Verification items for the finished model (mm, model axes). A direction names the side the tool comes from. Round coordinates to 2 decimals unless told otherwise and drop trailing zeros. Write item = value, one per line. Start each with the question number.
from build123d import *

# Parameters (mm, degrees)
SKETCH1_R                        = 45.085
BOSS_EXTRUDE1_DEPTH              = 9.525
SKETCH2_R                        = 41.402
BOSS_EXTRUDE2_DEPTH              = 7.1374
SKETCH3_R                        = 45.085
BOSS_EXTRUDE3_DEPTH              = 3.175
SKETCH4_R                        = 41.529
BOSS_EXTRUDE4_DEPTH              = 7.1374
SKETCH5_R                        = 45.085
BOSS_EXTRUDE5_DEPTH              = 3.175
CIRPATTERN1_COUNT                = 8
M10X1_0_TAPPED_HOLE1_D           = 9
M10X1_0_TAPPED_HOLE1_DEPTH       = 25
M10X1_0_TAPPED_HOLE1_CBORE_D     = 10
M10X1_0_TAPPED_HOLE1_CBORE_DEPTH = 20
M10X1_0_TAPPED_HOLE1_TIP         = 2.703872786
SKETCH9_R                        = 32.259
CUT_EXTRUDE1_DEPTH               = 21.2598
SKETCH11_R                       = 50.546
BOSS_EXTRUDE6_DEPTH              = 9.525
SKETCH12_R                       = 28.575
CUT_EXTRUDE2_DEPTH               = 9.525
F_15_0_18_DIAMETER_HOLE1_D       = 4.572
F_15_0_18_DIAMETER_HOLE1_DEPTH   = 9.525
CIRPATTERN2_COUNT                = 8


with BuildPart() as part:
    # Sketch1 → Boss-Extrude1 (new body)
    with BuildSketch(Plane(origin=(0, 0, 0), x_dir=(1, 0, 0), z_dir=(0, 1, 0))):
        with Locations(Location((0, 0, 0), (0, 0, 90))):
            Circle(SKETCH1_R)
    extrude(amount=BOSS_EXTRUDE1_DEPTH)

    # Sketch2 → Boss-Extrude2 (add)
    with BuildSketch(Plane(origin=(0, 9.525, 0), x_dir=(1, 0, 0), z_dir=(0, 1, 0))):
        with Locations(Location((0, 0, 0), (0, 0, 270))):
            Circle(SKETCH2_R)
    extrude(amount=BOSS_EXTRUDE2_DEPTH)

    # Sketch3 → Boss-Extrude3 (add)
    with BuildSketch(Plane(origin=(0, 16.6624, 0), x_dir=(1, 0, 0), z_dir=(0, 1, 0))):
        with Locations(Location((0, 0, 0), (0, 0, 90))):
            Circle(SKETCH3_R)
    extrude(amount=BOSS_EXTRUDE3_DEPTH)

    # Sketch4 → Boss-Extrude4 (add)
    with BuildSketch(Plane(origin=(0, 19.8374, 0), x_dir=(1, 0, 0), z_dir=(0, 1, 0))):
        with Locations(Location((0, 0, 0), (0, 0, 270))):
            Circle(SKETCH4_R)
    extrude(amount=BOSS_EXTRUDE4_DEPTH)

    # Sketch5 → Boss-Extrude5 (add)
    with BuildSketch(Plane(origin=(0, 26.9748, 0), x_dir=(1, 0, 0), z_dir=(0, 1, 0))):
        with Locations(Location((0, 0, 0), (0, 0, 90))):
            Circle(SKETCH5_R)
    extrude(amount=BOSS_EXTRUDE5_DEPTH)

    # Sketch6 → #15 (0.18) Diameter Hole2 (revolve, cut)
    with BuildSketch(Plane(origin=(-45.085, 4.7625, 0), x_dir=(0, 0, 1), z_dir=(0, 1, 0))):
        Polygon((0, 0), (0, 6.373567375), (2.286, 5), (2.286, 0), align=None)
    f_15_0_18_diameter_hole2 = revolve(axis=Axis((-51.435, 4.7625, 0), (1, 0, 0)), mode=Mode.SUBTRACT)

    # CirPattern1: #15 (0.18) Diameter Hole2 ×8 about axis
    cirpattern1_axis = Axis((0, 9.525, 0), (0, -1, 0))
    for i in range(1, CIRPATTERN1_COUNT):
        add(f_15_0_18_diameter_hole2.rotate(cirpattern1_axis, i * 360 / CIRPATTERN1_COUNT), mode=Mode.SUBTRACT)

    # M10x1.0 Tapped Hole1
    with Locations(Plane(origin=(0, 0, 0), x_dir=(-1, 0, 0), z_dir=(0, -1, 0))):
        with Locations((0, 0)):
            CounterBoreHole(M10X1_0_TAPPED_HOLE1_D / 2, M10X1_0_TAPPED_HOLE1_CBORE_D / 2, M10X1_0_TAPPED_HOLE1_CBORE_DEPTH, depth=M10X1_0_TAPPED_HOLE1_DEPTH)
            with Locations((0, 0, -(M10X1_0_TAPPED_HOLE1_DEPTH + M10X1_0_TAPPED_HOLE1_TIP / 2))):  # 118° drill point
                Cone(0, M10X1_0_TAPPED_HOLE1_D / 2, M10X1_0_TAPPED_HOLE1_TIP, mode=Mode.SUBTRACT)

    # Sketch9 → Cut-Extrude1 (cut)
    with BuildSketch(Plane(origin=(0, 30.1498, 0), x_dir=(1, 0, 0), z_dir=(0, 1, 0))):
        with Locations(Location((0, 0, 0), (0, 0, 270))):
            Circle(SKETCH9_R)
    extrude(amount=-CUT_EXTRUDE1_DEPTH, mode=Mode.SUBTRACT)

    # Sketch11 → Boss-Extrude6 (add)
    with BuildSketch(Plane(origin=(0, 0, 0), x_dir=(-1, 0, 0), z_dir=(0, -1, 0))):
        with Locations(Location((0, 0, 0), (0, 0, 270))):
            Circle(SKETCH11_R)
    extrude(amount=BOSS_EXTRUDE6_DEPTH)

    # Sketch12 → Cut-Extrude2 (cut)
    with BuildSketch(Plane.XZ.offset(9.525)):
        with Locations(Location((0, 0, 0), (0, 0, 270))):
            Circle(SKETCH12_R)
    extrude(amount=-CUT_EXTRUDE2_DEPTH, mode=Mode.SUBTRACT)

    # #15 (0.18) Diameter Hole1
    with Locations(Plane(origin=(15.459601618, -9.525, -43.838083818), x_dir=(0, 0, -1), z_dir=(0, -1, 0))):
        with Locations((0, 0)):
            f_15_0_18_diameter_hole1 = Hole(F_15_0_18_DIAMETER_HOLE1_D / 2, depth=F_15_0_18_DIAMETER_HOLE1_DEPTH)

    # CirPattern2: #15 (0.18) Diameter Hole1 ×8 about axis
    cirpattern2_axis = Axis((0, 0, 0), (0, 1, 0))
    for i in range(1, CIRPATTERN2_COUNT):
        add(f_15_0_18_diameter_hole1.rotate(cirpattern2_axis, i * 360 / CIRPATTERN2_COUNT), mode=Mode.SUBTRACT)


solid = part.part
(1) Set-up check for faces 1 (the flat face through (45, 0, -8)), 2 (the cylindrical face through (19.36, -4.7, 46.69)), 3 (the cylindrical face through (46.12, -4.7, 15.56)), 4 (the conical face through (27.82, 4.75, -27.26)): record each of +Z, -Z, +X, -X, +Y, -Y from which the full face is reachable in a straight line by a thin tool's end or side.
(2) Depth check by flat-ended pin: pin 1 (5 mm diameter, centred on x = -17, y = 25.5, fed in from +Z); pin 2 (4 mm diameter, centred on x = 28, y = 1.5, fed in from -Z); pin 3 (2.5 mm diameter, centred on x = 0, y = 4.76, fed in from +Z). Enter the tip coordinate at first touch or a pass-through.
(3) Scan lines: line 1 along X through (y, z) = (-1.75, 0) (3 decimals); line 2 along Y through (x, z) = (-26, 34.5) (3 decimals); line 3 along Y through (x, z) = (-42, 0) (1 decimal). Record each from-to range of solid material in increasing order. Write a range as from..to.
(4) Draft check along Z on faces 5 (the cylindrical face through (1.229, 2.835, 42.62)), 6 (the cylindrical face through (44.013, 28.54, 9.774)), 7 (the conical face through (-38.95, 5.15, -0.09)), 8 (the cylindrical face through (15.56, -4.7, -46.12)). Enter one of: +Z half, -Z half, draft (parallel to the pull), parting line (faces both ways), or undercut.
Outcome:
q1.face_1 = +Y
q1.face_2 = +Y, -Y
q1.face_3 = -Y
q1.face_4 = none
q2.pin_1 = 42.52
q2.pin_2 = -42.93
q2.pin_3 = 39.46
q3.line_1 = -50.546..-28.575, 28.575..50.546
q3.line_2 = -9.525..9.525, 16.662..19.837, 26.975..30.15
q3.line_3 = -9.5..2.5, 7..9.5, 16.7..19.8, 27..30.1
q4.face_5 = draft
q4.face_6 = parting line
q4.face_7 = undercut
q4.face_8 = undercut
